from build123d import *

# Parameters (mm, degrees)
BOSS_EXTRUDE1_DEPTH = 10
FILLET11_R          = 5
FILLET12_R          = 5
FILLET13_R          = 5
SKETCH7_W           = 10
SKETCH7_H           = 2
BOSS_EXTRUDE5_DEPTH = 10
SKETCH8_W           = 10
SKETCH8_H           = 2
BOSS_EXTRUDE6_DEPTH = 10
SKETCH9_R           = 2.5
CUT_EXTRUDE2_DEPTH  = 10


with BuildPart() as part:
    # Sketch2 → Boss-Extrude1 (new body)
    with BuildSketch(Plane.XY):
        with BuildLine():
            Line((24.5, -20.5), (32.5, -20.5))
            Line((32.5, -20.5), (32.5, -22.5))
            Line((32.5, -22.5), (22.5, -22.5))
            Line((22.5, -22.5), (22.5, 0))
            ThreePointArc((22.5, 0), (0, 22.5), (-22.5, 0))
            Line((-22.5, 0), (-22.5, -22.5))
            Line((-22.5, -22.5), (-32.5, -22.5))
            Line((-32.5, -22.5), (-32.5, -20.5))
            Line((-32.5, -20.5), (-24.5, -20.5))
            Line((-24.5, -20.5), (-24.5, 0))
            ThreePointArc((-24.5, 0), (0, 24.5), (24.5, 0))
            Line((24.5, 0), (24.5, -20.5))
        make_face()
    extrude(amount=BOSS_EXTRUDE1_DEPTH)

    # Fillet11
    fillet11_edges = [part.edges().sort_by_distance(p)[0] for p in [
        (-22.5, -22.5, 5),
    ]]
    fillet(fillet11_edges, radius=FILLET11_R)

    # Fillet12
    fillet12_edges = [part.edges().sort_by_distance(p)[0] for p in [
        (-24.5, -20.5, 5),
    ]]
    fillet(fillet12_edges, radius=FILLET12_R)

    # Fillet13
    fillet13_edges = [part.edges().sort_by_distance(p)[0] for p in [
        (24.5, -20.5, 5),
        (22.5, -22.5, 5),
    ]]
    fillet(fillet13_edges, radius=FILLET13_R)

    # Sketch7 → Boss-Extrude5 (add)
    with BuildSketch(Plane(origin=(32.5, 0, 0), x_dir=(0, 0, -1), z_dir=(1, 0, 0))):
        with Locations((-5, -21.5)):
            Rectangle(SKETCH7_W, SKETCH7_H)
    extrude(amount=BOSS_EXTRUDE5_DEPTH)

    # Sketch8 → Boss-Extrude6 (add)
    with BuildSketch(Plane.ZY.offset(32.5)):
        with Locations((5, -21.5)):
            Rectangle(SKETCH8_W, SKETCH8_H)
    extrude(amount=BOSS_EXTRUDE6_DEPTH)

    # Sketch9 → Cut-Extrude2 (cut)
    with BuildSketch(Plane(origin=(0, -20.5, 0), x_dir=(1, 0, 0), z_dir=(0, 1, 0))):
        with Locations(Location((-35, -5, 0), (0, 0, 180))):
            Circle(SKETCH9_R)
    cut_extrude2 = extrude(amount=-CUT_EXTRUDE2_DEPTH, mode=Mode.SUBTRACT)

    # Mirror2: Cut-Extrude2 across plane
    add(cut_extrude2.mirror(Plane(origin=(0, 0, 0), x_dir=(0, 0, 1), z_dir=(1, 0, 0))), mode=Mode.SUBTRACT)


solid = part.part
Geometry: final body of the model. Coordinates: model frame, mm. A direction names the side the tool comes from. Round coordinates to 2 decimals unless told otherwise and drop trailing zeros. Loops run counter-clockwise (first coordinate to the right, second up) from the corner with the lowest first, then second, coordinate; pieces in that order, holes last. Notation, with made-up numbers: M 45.25,78 L 69.25,78 A19 cw 69.25,83 Z; hole C 74,-36 d4. An arc over 180 degrees is marked long. Put each result on its own line as item: value. Start each with the question number.
(1) Section query C-C (y = -4.5). Return loops of the section in (x, z), then the cut area to 3 significant figures.
(2) Section query D-D (x = 0). Return loops of the section in (y, z), then the cut area to 3 significant figures.
(3) Section query A-A (z = 5). Return loops of the section in (x, y), then the cut area to 3 significant figures.
(4) Section query B-B (x = -35). Return loops of the section in (y, z).
(5) Material intervals for line 1 along Z through (x, y) = (-35, -21.9); line 2 along X through (y, z) = (-15.5, 5.5); line 3 along X through (y, z) = (14, 8), sorted ascending. Write a range as [from, to].
(6) Contact query for flat-ended pins moving along their axis: pin 1 Ø5 at (y, z) = (-8.5, 3.5) entering from +X; pin 2 Ø6 at (x, z) = (35, 5) entering from +Y; pin 3 Ø1.5 at (y, z) = (15.5, 4) entering from +X. Output: stop coordinate, or through.
(7) Set-up query: faces 5 (the face through (37.4, -20.5, 6.2)), 6 (the face through (-24.5, -8, 5)), 7 (the face through (23.93, -21, 5.07)). Return all of +Z, -Z, +X, -X, +Y, -Y with unobstructed straight access to the full face (end or side cutting, diameter ignored); none if empty.
(8) Draft query along X for faces 1 (the face through (42.5, -21, 5)), 2 (the face through (0.495, 22.495, 4.93)), 3 (the face through (33, -22.5, 3)), 4 (the face through (-23.93, -21, 5.07)). Return one class per face: +X half, -X half, draft (parallel to the pull), parting line (faces both ways), or undercut.
Findings below:
1. outline: M -24.5,0 L -22.5,0 L -22.5,10 L -24.5,10 Z; M 22.5,0 L 24.5,0 L 24.5,10 L 22.5,10 Z
1. area: 40.0 mm2
2. outline: M 22.5,0 L 24.5,0 L 24.5,10 L 22.5,10 Z
2. area: 20.0 mm2
3. outline: M -42.5,-22.5 L -37.5,-22.5 L -37.5,-20.5 L -42.5,-20.5 Z; M -32.5,-22.5 L -27.5,-22.5 A5 ccw -22.5,-17.5 L -22.5,0 A22.5 cw 22.5,0 L 22.5,-17.5 A5 ccw 27.5,-22.5 L 32.5,-22.5 L 32.5,-20.5 L 29.5,-20.5 A5 cw 24.5,-15.5 L 24.5,0 A24.5 ccw -24.5,0 L -24.5,-15.5 A5 cw -29.5,-20.5 L -32.5,-20.5 Z; M 37.5,-22.5 L 42.5,-22.5 L 42.5,-20.5 L 37.5,-20.5 Z
3. area: 290 mm2
4. outline: M -22.5,0 L -20.5,0 L -20.5,2.5 L -22.5,2.5 Z; M -22.5,7.5 L -20.5,7.5 L -20.5,10 L -22.5,10 Z
5. line 1: z = [0, 2.5], [7.5, 10]
5. line 2: x = [-24.5, -22.5], [22.5, 24.5]
5. line 3: x = [-20.11, -17.61], [17.61, 20.11]
6. pin 1: stops at x = 24.5
6. pin 2: stops at y = -20.5
6. pin 3: stops at x = 19.56
7. face 5: +Z, -Z, +X, +Y
7. face 6: +Z, -Z, -X, +Y
7. face 7: +Z, -Z, -Y
8. face 1: +X half
8. face 2: undercut
8. face 3: draft
8. face 4: undercut
